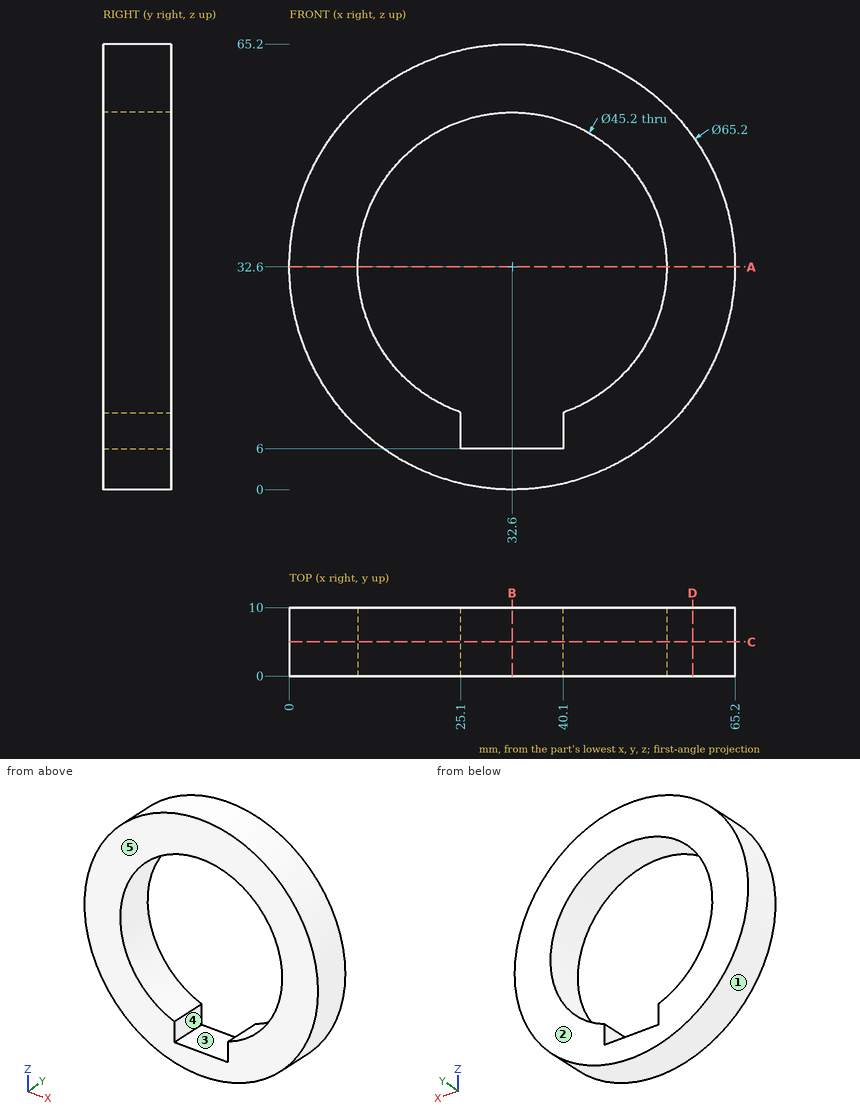
Geometry: see drawing. Coordinates: mm, zero at the bounding-box minimum. A direction names the side the tool comes from. Give positions to 0.01 mm unless a question says otherwise; leave off trailing zeros. Write each loop counter-clockwise with the first axis right and the second up, starting at its lowest first coordinate (ties: lowest second). Pieces come first, ordered by that corner, then holes. Notation, with made-up numbers: M 67.25,25 L 89.25,25 A19 ccw 89.25,38 Z; hole C -13.5,69 d2. An arc over 180 degrees is marked long. Answer in a Markdown table with one row per item. Add a question column.
(1) Section B-B on x = 32.6. Return loops of the section in (y, z), and give its area (3 significant figures).
(2) Section A-A on z = 32.6. Return loops of the section in (x, y), and give its area (3 significant figures).
(3) First-contact query: pin 1 (1 mm diameter, centred on y = 2, z = 23, fed in from +X); pin 2 (4 mm diameter, centred on y = 3.5, z = 8.5, fed in from +X); pin 3 (4 mm diameter, centred on y = 5.5, z = 8.5, fed in from -X). Flat tips, straight axial feed; report the tip coordinate or a pass-through.
(4) Section D-D on x = 59. Return loops of the section in (y, z), and give its area (3 significant figures).
(5) Ray query, line 1 (Z direction, x = 32.6, y = 7.75); line 2 (X direction, y = 5.75, z = 33); line 3 (X direction, y = 2.5, z = 38.5). Return the intervals inside material, ascending.
(6) Mould query, pull axis X, two halves, no side actions, for the marked faces 1, 2 and 3. Classes: +X half, -X half, draft (parallel to the pull), parting line (faces both ways), or undercut.
(7) Section C-C on y = 5. Return loops of the section in (x, z).
(8) Reachability of the marked faces 4 and 5 from +Z, -Z, +X, -X, +Y, -Y: full face, straight path, thin tool, end or side. Return the list, or none.
Result set:
| question | item | result |
|---|---|---|
| 1 | outline | M 0,0 L 10,0 L 10,6 L 0,6 Z; M 0,55.2 L 10,55.2 L 10,65.2 L 0,65.2 Z |
| 1 | area | 160 mm^2 |
| 2 | outline | M 0,0 L 10,0 L 10,10 L 0,10 Z; M 55.2,0 L 65.2,0 L 65.2,10 L 55.2,10 Z |
| 2 | area | 200 mm^2 |
| 3 | pin 1 | stops at x = 63.9 |
| 3 | pin 2 | stops at x = 56.57 |
| 3 | pin 3 | stops at x = 8.63 |
| 4 | outline | M 0,13.47 L 10,13.47 L 10,51.73 L 0,51.73 Z |
| 4 | area | 383 mm^2 |
| 5 | line 1 | z = 0 to 6, 55.2 to 65.2 |
| 5 | line 2 | x = 0 to 10, 55.2 to 65.2 |
| 5 | line 3 | x = 0.54 to 10.78, 54.42 to 64.66 |
| 6 | face 1 | parting line |
| 6 | face 2 | draft |
| 6 | face 3 | undercut |
| 7 | outline | C 32.6,32.6 d65.2; hole M 25.1,6 L 40.1,6 L 40.1,11.28 A22.6 ccw long 25.1,11.28 Z |
| 8 | face 4 | +Y, -Y |
| 8 | face 5 | +Z, -Z, +X, -X, -Y |
